Read the model definition and answer for the solid it produces. Units are mm, in the model's axes. Face numbers are marked on the shaded views. Round coordinates to 2 decimals unless told otherwise and drop trailing zeros. Order: outer loops, then holes, each group sorted by start corner. A loop starts at its lowest first (then second) coordinate and runs counter-clockwise, first axis right, second up. Notation, with made-up numbers: (41, 78) - (82, 78) arc R22 cw to (82, 94) - close; hole circle Ø7 at (87, 73.5). An arc over 180 degrees is marked (long way). Answer as a JSON object with one key per item and string values. Group by question number.
Q1. A cutting plane is placed at C-C on z = 0.5. Determine the outline of the cut face in (x, y).
Q2. Consider line 1 (Z direction, x = -16.5, y = -2.15); line 2 (Z direction, x = -16.75, y = -3.7); line 3 (X direction, y = -1.8, z = -1.5). Determine where each line is inside the solid, lowest interval first.
Q3. The mould has two halves that part along Z. Classify the marked faces 1, 2 and 3: pulls with the +Z half, pulls with the -Z half, needs draft (parallel to the pull), parting line crosses it, or undercut.
Q4. A cutting plane is placed at D-D on x = -24.5. Determine the outline of the cut face in (y, z).
Q5. Given pin 1 Ø1.5 at (x, z) = (-16.5, 1) entering from -Y; pin 2 Ø1 at (y, z) = (-2.5, 3) entering from +X, each flat-ended and moving along its own axis, determine where each tip first touches the part or whether it passes through.
Q6. A cutting plane is placed at A-A on z = 6.75. Determine the outline of the cut face in (x, y), and give its area (3 significant figures).
Q7. A cutting plane is placed at B-B on x = -17.25. Determine the outline of the cut face in (y, z), and give its area (3 significant figures).
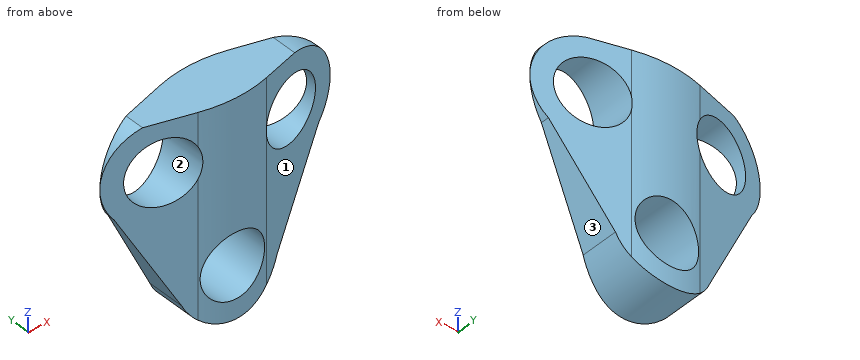
```python
from build123d import *

# Parameters (mm, degrees)
F0_R     = 2.5
F1_DEPTH = 5
F2_DEPTH = 7.6
F4_DEPTH = 12.5


with BuildPart() as f1:
    # F0 (on Front) → F1 (new body)
    with BuildSketch(Plane.XZ):
        with BuildLine():
            ThreePointArc((-13.985505, -0.040325), (-18.794733, 3.876963), (-21.658079, -1.625316))
            ThreePointArc((-21.658079, -1.625316), (-17.895778, -4.039319), (-14.245536, -1.458999))
            ThreePointArc((-14.245536, -1.458999), (-14.05105, -0.761479), (-13.985505, -0.040325))
        make_face()
        with Locations((-17.985505, -0.040325)):
            Circle(F0_R, mode=Mode.SUBTRACT)
        with BuildLine():
            ThreePointArc((-8.813406, 8.51826), (-9.956912, 11.31834), (-12.733627, 12.517465))
            ThreePointArc((-12.733627, 12.517465), (-16.526603, 7.030925), (-9.994852, 5.679994))
            ThreePointArc((-9.994852, 5.679994), (-9.12056, 6.98109), (-8.813406, 8.51826))
        make_face()
        with Locations((-12.813406, 8.51826)):
            Circle(F0_R, mode=Mode.SUBTRACT)
        with Locations((-17.985505, -0.040325)):
            Circle(F0_R)
        with Locations((-12.813406, 8.51826)):
            Circle(F0_R)
        with Locations((-22.811408, 8.718137)):
            Circle(F0_R)
        with BuildLine():
            ThreePointArc((-22.673007, 12.715742), (-19.934465, 11.497201), (-18.811408, 8.718137))
            ThreePointArc((-18.811408, 8.718137), (-21.464184, 4.951841), (-25.903902, 6.181114))
            Line((-25.903902, 6.181114), (-21.658079, -1.625316))
            ThreePointArc((-21.658079, -1.625316), (-18.794733, 3.876963), (-13.985505, -0.040325))
            ThreePointArc((-13.985505, -0.040325), (-14.05105, -0.761479), (-14.245536, -1.458999))
            Line((-14.245536, -1.458999), (-9.994852, 5.679994))
            ThreePointArc((-9.994852, 5.679994), (-16.526603, 7.030925), (-12.733627, 12.517465))
            Line((-12.733627, 12.517465), (-22.673007, 12.715742))
        make_face()
        with BuildLine():
            ThreePointArc((-25.903902, 6.181114), (-21.464184, 4.951841), (-18.811408, 8.718137))
            ThreePointArc((-18.811408, 8.718137), (-19.934465, 11.497201), (-22.673007, 12.715742))
            ThreePointArc((-22.673007, 12.715742), (-26.397075, 10.490986), (-25.903902, 6.181114))
        make_face()
        with Locations((-22.811408, 8.718137)):
            Circle(F0_R, mode=Mode.SUBTRACT)
    extrude(amount=F1_DEPTH)

    # F0 (on Front) → F2 (cut)
    with BuildSketch(Plane.XZ):
        with Locations((-22.811408, 8.718137)):
            Circle(F0_R)
        with Locations((-12.813406, 8.51826)):
            Circle(F0_R)
        with Locations((-17.985505, -0.040325)):
            Circle(F0_R)
    extrude(amount=F2_DEPTH, mode=Mode.SUBTRACT)

    # F3 (on Top) → F4 (intersect, symmetric)
    with BuildSketch(Plane.XY):
        with BuildLine():
            Line((-26.811408, -2.5), (-20.626082, -4.245374))
            ThreePointArc((-20.626082, -4.245374), (-17.950294, -4.621121), (-15.271588, -4.26677))
            Line((-15.271588, -4.26677), (-8.813406, -2.5))
            Line((-8.813406, -2.5), (-15.271588, -0.73323))
            ThreePointArc((-15.271588, -0.73323), (-17.950294, -0.378879), (-20.626082, -0.754626))
            Line((-20.626082, -0.754626), (-26.811408, -2.5))
        make_face()
    extrude(amount=F4_DEPTH, both=True, mode=Mode.INTERSECT)


solid = f1.part
```
Result set:
{
 "1": {"outline": "(-22.81, -3.63) - (-20.63, -4.25) arc R10 ccw to (-20.43, -4.3) - (-20.43, -0.7) arc R10 ccw to (-20.63, -0.75) - (-22.81, -1.37) - close; (-15.54, -4.34) arc R10 ccw to (-15.27, -4.27) - (-13.08, -3.67) - (-13.08, -1.33) - (-15.27, -0.73) arc R10 ccw to (-15.54, -0.66) - close"},
 "2": {"line 1": "z = -3.75 to -2.05, 1.97 to 12.5", "line 2": "z = -3.84 to -2.21, 2.13 to 12.5", "line 3": "x = -21.73 to -20.02, -15.96 to -14.26"},
 "3": {"face 1": "needs draft", "face 2": "undercut", "face 3": "pulls with the -Z half"},
 "4": {"outline": "(-3.15, 3.6) - (-1.85, 3.6) - (-1.85, 6.87) - (-3.15, 6.87) - close; (-3.15, 10.56) - (-1.85, 10.56) - (-1.85, 12.34) - (-3.15, 12.34) - close"},
 "5": {"pin 1": "stops at y = -4.47", "pin 2": "stops at x = -11.29"},
 "6": {"outline": "(-26.29, -2.65) - (-24.35, -3.19) - (-24.35, -1.81) - (-26.29, -2.35) - close; (-21.27, -4.06) - (-20.63, -4.25) arc R10 ccw to (-15.27, -4.27) - (-14.58, -4.08) - (-14.58, -0.92) - (-15.27, -0.73) arc R10 ccw to (-20.63, -0.75) - (-21.27, -0.94) - close; (-11.05, -3.11) - (-9.23, -2.61) - (-9.23, -2.39) - (-11.05, -1.89) - close", "area": "28.8 mm²"},
 "7": {"outline": "(-4.6, -3.97) - (-0.4, -3.97) - (-0.4, -2.43) - (-4.6, -2.43) - close; (-4.6, 2.35) - (-0.4, 2.35) - (-0.4, 12.5) - (-4.6, 12.5) - close", "area": "49.1 mm²"}
}
